Model file for the job. Use its own axes, mm. A direction names the side the tool comes from. Give positions to 0.01 mm unless a question says otherwise; leave off trailing zeros. Order: outer loops, then holes, each group sorted by start corner. A loop starts at its lowest first (then second) coordinate and runs counter-clockwise, first axis right, second up. Notation, with made-up numbers: (23, 27.25) - (27, 27.25) arc R27 ccw to (27, 54.25) - close; hole circle Ø1 at (52, 80.5). An arc over 180 degrees is marked (long way). Use CSV: the item, a comma, the result in double quotes. Start each with the question number.
(1) Drop a flat-ended pin along its axis: pin 1 Ø2.5 at (x, y) = (49.5, 1.5) entering from -Z. Give the stop position or say it passes through.
(2) Band-saw the part on D-D, the plane z = 35. Give the cut face in (x, y) (3 decimals).
(3) Band-saw the part on B-B, the plane z = 64. Give the cut face in (x, y) (3 decimals), then the cut area to 3 significant figures.
(4) Pull direction X, two halves, no side cores. Call faces 1 (the flat face through (47.625, -1, 64)), 2 (the flat face through (-50.8, -1, 64)), 3 (the flat face through (-1, -50.8, 64)): +X half, -X half, draft (parallel to the pull), parting line (faces both ways), or undercut.
(5) Probe L1, parallel to Y at x = 9, z = 84 (3 decimals); L2, parallel to X at y = 7, z = 64 (3 decimals). List the from-to ranges inside material, lowest first.
(6) Band-saw the part on A-A, the plane y = -23. Give the cut face in (x, z) (3 decimals).
(7) Tool access for faces 4 (the cylindrical face through (49.23, -8.85, 116.78)), 5 (the flat face through (50.8, 0, 64)), 6 (the flat face through (-47.625, -1, 64)): list every direction of +Z, -Z, +X, -X, +Y, -Y with a clear straight run to the whole face (end or side of a thin tool).
from build123d import *

# Parameters (mm, degrees)
F0_W     = 101.6
F0_H     = 101.6
F0_W_2   = 95.25
F0_H_2   = 95.25
F1_DEPTH = 130
F2_R     = 2
F3_W     = 6.54
F3_H     = 9.4
F4_DEPTH = 3.175
F5_R     = 2.6666666667
F6_DEPTH = 1.27


# Not quite as in the source:
# - a length typed as a fraction of an inch, garbled in the dataset ("3 / 203.2 mm" for 3/8 in), is restored


with BuildPart() as f1:
    # F0 (on Top) → F1 (new body)
    with BuildSketch(Plane.XY):
        Rectangle(F0_W, F0_H)
        Rectangle(F0_W_2, F0_H_2, mode=Mode.SUBTRACT)
    extrude(amount=F1_DEPTH)

    # F2
    f2_edges = [f1.edges().sort_by_distance(p)[0] for p in [
        (50.8, 50.8, 65),
        (-50.8, 50.8, 65),
        (50.8, -50.8, 65),
        (-50.8, -50.8, 65),
    ]]
    fillet(f2_edges, radius=F2_R)

    # F3 (on face) → F4 (cut)
    with BuildSketch(Plane.YZ.offset(50.8)):
        with Locations((-3.27, 116.7)):
            Rectangle(F3_W, F3_H)
        with BuildLine():
            Line((-6.54, 112), (-6.54, 121.4))
            ThreePointArc((-6.54, 121.4), (-8.85, 116.7), (-6.54, 112))
        make_face()
        with Locations((3.27, 116.7)):
            Rectangle(F3_W, F3_H)
        with BuildLine():
            ThreePointArc((6.54, 112), (8.85, 116.7), (6.54, 121.4))
            Line((6.54, 121.4), (6.54, 112))
        make_face()
        with BuildLine():
            Line((0, 84), (0, 100))
            ThreePointArc((0, 100), (-8, 92), (0, 84))
        make_face()
        with BuildLine():
            ThreePointArc((8, 92), (5.6568542495, 97.6568542495), (0, 100))
            Line((0, 100), (0, 84))
            ThreePointArc((0, 84), (5.6568542495, 86.3431457505), (8, 92))
        make_face()
    extrude(amount=-F4_DEPTH, mode=Mode.SUBTRACT)

    # F5 (on face) → F6 (cut)
    with BuildSketch(Plane.YZ.offset(50.8)):
        with BuildLine():
            Line((0, 84), (0, 100))
            ThreePointArc((0, 100), (-8, 92), (0, 84))
        make_face()
        with BuildLine():
            ThreePointArc((8, 92), (5.6568542495, 97.6568542495), (0, 100))
            Line((0, 100), (0, 84))
            ThreePointArc((0, 84), (5.6568542495, 86.3431457505), (8, 92))
        make_face()
        with BuildLine():
            ThreePointArc((-3.4833400656, 71.2018290724), (-3.7712361663, 67.7712361663), (-7.2018290724, 67.4833400656))
            ThreePointArc((-7.2018290724, 67.4833400656), (-8, 64), (-7.2018290724, 60.5166599344))
            ThreePointArc((-7.2018290724, 60.5166599344), (-3.7712361663, 60.2287638337), (-3.4833400656, 56.7981709276))
            ThreePointArc((-3.4833400656, 56.7981709276), (0, 56), (3.4833400656, 56.7981709276))
            ThreePointArc((3.4833400656, 56.7981709276), (3.7712361663, 60.2287638337), (7.2018290724, 60.5166599344))
            ThreePointArc((7.2018290724, 60.5166599344), (8, 64), (7.2018290724, 67.4833400656))
            ThreePointArc((7.2018290724, 67.4833400656), (3.7712361663, 67.7712361663), (3.4833400656, 71.2018290724))
            ThreePointArc((3.4833400656, 71.2018290724), (0, 72), (-3.4833400656, 71.2018290724))
        make_face()
        with Locations((0, 64)):
            Circle(F5_R, mode=Mode.SUBTRACT)
    extrude(amount=-F6_DEPTH, mode=Mode.SUBTRACT)


solid = f1.part
Answer block:
1,pin 1,"stops at z = 0"
2,outline,"(-50.8, -48.8) arc R2 ccw to (-48.8, -50.8) - (48.8, -50.8) arc R2 ccw to (50.8, -48.8) - (50.8, 48.8) arc R2 ccw to (48.8, 50.8) - (-48.8, 50.8) arc R2 ccw to (-50.8, 48.8) - close; hole (-47.625, -47.625) - (47.625, -47.625) - (47.625, 47.625) - (-47.625, 47.625) - close"
3,outline,"(-50.8, -48.8) arc R2 ccw to (-48.8, -50.8) - (48.8, -50.8) arc R2 ccw to (50.8, -48.8) - (50.8, -8) - (49.53, -8) - (49.53, -2.667) - (50.8, -2.667) - (50.8, 2.667) - (49.53, 2.667) - (49.53, 8) - (50.8, 8) - (50.8, 48.8) arc R2 ccw to (48.8, 50.8) - (-48.8, 50.8) arc R2 ccw to (-50.8, 48.8) - close; hole (-47.625, -47.625) - (47.625, -47.625) - (47.625, 47.625) - (-47.625, 47.625) - close"
3,area,"1,230 mm2"
4,face 1,"undercut"
4,face 2,"-X half"
4,face 3,"draft"
5,L1,"y = -50.8 to -47.625, 47.625 to 50.8"
5,L2,"x = -50.8 to -47.625, 47.625 to 49.53"
6,outline,"(-50.8, 0) - (-47.625, 0) - (-47.625, 130) - (-50.8, 130) - close; (47.625, 0) - (50.8, 0) - (50.8, 130) - (47.625, 130) - close"
7,face 4,"+X"
7,face 5,"+Z, -Z, +X, +Y, -Y"
7,face 6,"+Z, -Z"
